Source: CAD feature listing. Evaluate the final solid. Frame: model axes, mm. Coordinates: 2 decimals unless noted, no trailing zeros. One line per item, written item: value. Start each with the question number.
1. Mould query, pull axis X, two halves, no side actions, for faces 1 (the cylindrical face through (2.904, -0.166, 0.815)), 2 (the flat face through (0.7, -11, 2.7)), 3 (the cylindrical face through (0.9, -0.15, 0.86)), 4 (the flat face through (15.74, 0.65, 2.37)). Classes: released by +X, released by -X, zero draft, split by the parting line, or undercut.
2. First-contact query: P1, Ø10, axis at x = 5.5, y = 5, coming from the -Z side; P2, Ø10, axis at x = 18, y = 6.5, coming from the -Z side; P3, Ø1, axis at x = 9, y = 0, coming from the -Z side; P4, Ø5, axis at x = 18.5, y = 3.5, coming from the +Z side. Flat tips, straight axial feed; report the tip coordinate or a pass-through.
3. Line query: line 1 (Z direction, x = 3.5, y = 1.25); line 2 (X direction, y = 0, z = 3.5); line 3 (X direction, y = 7.75, z = 3.25). Output: solid intervals per line, ascending.
4. Section query A-A, the plane y = 0. State how many separate pieces and enclosed holes the cut face has, and give its area (3 significant figures).
from build123d import *

# Parameters (mm, degrees)
F0_R         = 0.75
F1_DEPTH     = 7
F2_R         = 2.75
F3_DEPTH     = 25
F4_R         = 3
F6_DEPTH     = 25
F7_R         = 1.5
F8_DEPTH     = 0.5
F9_R         = 1.5
F10_DEPTH    = 0.5
F11_T4_DEPTH = 19.1627380087


# Not quite as in the source:
# - a fillet or chamfer that OpenCascade refuses, or shapes differently, is made with other operations: its cross-section is extruded or revolved along the edge and cut away or added


with BuildPart() as f1:
    # F0 (on Top) → F1 (new body)
    with BuildSketch(Plane.XY):
        with BuildLine():
            add(Edge.make_bspline(
                [(0, 11), (5.2254716866, 10.975911282), (20.5224081874, 7.3522534221), (22.6636249572, -4.0898798034)],
                knots=[0, 0, 0, 0, 27.2276397927, 27.2276397927, 27.2276397927, 27.2276397927], degree=3))
            Line((0, 11), (0, -11))
            Line((0, -11), (7, -11))
            add(Edge.make_bspline(
                [(7, -11), (10.2693928853, -5.7117650285), (14.8583007976, -2.8734656516), (22.6636249572, -4.0898798034)],
                knots=[0, 0, 0, 0, 17.1201316564, 17.1201316564, 17.1201316564, 17.1201316564], degree=3))
        make_face()
        with Locations((16.5, 0)):
            Circle(F0_R, mode=Mode.SUBTRACT)
    extrude(amount=F1_DEPTH)

    # F2 (on face) → F3 (cut)
    with BuildSketch(Plane.XZ.offset(11)):
        with Locations((3.5, 3.5)):
            Circle(F2_R)
    extrude(amount=-F3_DEPTH, mode=Mode.SUBTRACT)

    # F4
    f4_edges = [f1.edges().sort_by_distance(p)[0] for p in [
        (0, 0, 0),
        (0, 0, 7),
    ]]
    fillet(f4_edges, radius=F4_R)

    # F5 (on face) → F6 (cut)
    with BuildSketch(Plane.XZ.offset(11)):
        Polygon((7, 6.5709358384), (22.6717181504, 4), (26.1740684509, 7.8573133796), (11.5607753396, 11.3733848557), (4.3845428154, 7), (7, 7), align=None)
        Polygon((26.1740684509, -0.8573133796), (22.6717181504, 3), (7, 0.4290641616), (7, 0), (4.3845428154, 0), (11.5607753396, -4.3733848557), align=None)
        Polygon((4.3845428154, 7), (7, 6.5709358384), (7, 7), align=None)
        Polygon((7, 0), (7, 0.4290641616), (4.3845428154, 0), align=None)
    extrude(amount=-F6_DEPTH, mode=Mode.SUBTRACT)

    # F7 (on face) → F8 (cut)
    with BuildSketch(Plane(origin=(1.2331564946, 0, 7.5169830107), x_dir=(0.9868095474, 0, -0.1618855065), z_dir=(0.1618855065, 0, 0.9868095474))):
        with Locations((15.4709118351, 0)):
            Circle(F7_R)
    extrude(amount=-F8_DEPTH, mode=Mode.SUBTRACT)

    # F9 (on face) → F10 (cut)
    with BuildSketch(Plane(origin=(0.1149053506, 0, -0.7004314313), x_dir=(0.9868095474, 0, 0.1618855065), z_dir=(0.1618855065, 0, -0.9868095474))):
        with Locations((16.6041103809, 0)):
            Circle(F9_R)
    extrude(amount=-F10_DEPTH, mode=Mode.SUBTRACT)

    # F11: fillet of radius 5 on 1 edges, made by hand


with BuildPart() as f11_tool2:
    # F11_s3 → F11_t4 (new body)
    with BuildSketch(Plane.XY.offset(-6.0813690043)):
        with BuildLine():
            ThreePointArc((8.3278164384, -9.0886011335), (6.5818041274, -10.4968325334), (4.3958267336, -11))
            Line((4.3958267336, -11), (4.3958267336, -11.1))
            Line((4.3958267336, -11.1), (7, -11.1))
            Line((7, -11.1), (7.0850572831, -11.0525857262))
            ThreePointArc((7.0850572831, -11.0525857262), (7.7193199568, -10.0826857854), (8.4064562325, -9.1503731561))
            Line((8.4064562325, -9.1503731561), (8.3278164384, -9.0886011335))
        make_face()
    extrude(amount=F11_T4_DEPTH)

    split(bisect_by=Plane(origin=(0.1149053506, 0, -0.7004314313), x_dir=(0, 1, 0), z_dir=(-0.1618855065, 0, 0.9868095474)), keep=Keep.TOP)

    split(bisect_by=Plane(origin=(1.2331564946, 0, 7.5169830107), x_dir=(0, 1, 0), z_dir=(-0.1618855065, 0, -0.9868095474)), keep=Keep.TOP)


with BuildPart() as f1_1:
    add(f1.part)

    # F11_t1: cut F11_tool2
    add(f11_tool2.part, mode=Mode.SUBTRACT)


solid = f1_1.part
Computed values:
1. face 1: undercut
1. face 2: zero draft
1. face 3: released by -X
1. face 4: undercut
2. P1: stops at z = 0
2. P2: stops at z = 1.41
2. P3: stops at z = 0.68
2. P4: stops at z = 5.09
3. line 1: z = 0 to 0.75, 6.25 to 7
3. line 2: x = 0 to 0.75, 6.25 to 15.75, 17.25 to 21.2
3. line 3: x = 0 to 0.76, 6.24 to 12.46
4. separate pieces: 2
4. enclosed holes: 1
4. area: 68.4 mm²
